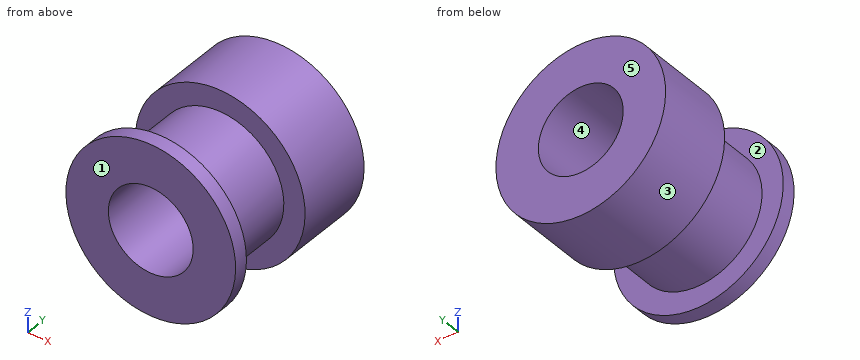
from build123d import *

# Parameters (mm, degrees)
SKETCH_1_R          = 8
EXTRUDE_1_DEPTH     = 1.35
SKETCH_4_R          = 6
EXTRUDE_3_DEPTH     = 7.3
EXTRUDE_START       = 8.65
SKETCH_1_3_R        = 8
EXTRUDE_4_DEPTH     = 7.35
SKETCH_5_R          = 4
CUT_EXTRUDE_1_DEPTH = 20.595917942


with BuildPart() as part:
    # 草图1 → 凸台-拉伸1 (new body)
    with BuildSketch(Plane(origin=(0, 0, 0), x_dir=(1, 0, 0), z_dir=(0, 1, 0))):
        with Locations(Location((0, 0, 0), (0, 0, 90))):
            Circle(SKETCH_1_R)
    extrude(amount=EXTRUDE_1_DEPTH)

    # 草图4 → 凸台-拉伸3 (add)
    with BuildSketch(Plane(origin=(0, 1.35, 0), x_dir=(1, 0, 0), z_dir=(0, 1, 0))):
        with Locations(Location((0, 0, 0), (0, 0, 270))):
            Circle(SKETCH_4_R)
    extrude(amount=EXTRUDE_3_DEPTH)

    # 草图1<3> → 凸台-拉伸4 (add)
    with BuildSketch(Plane(origin=(0, 0, 0), x_dir=(1, 0, 0), z_dir=(0, 1, 0)).offset(EXTRUDE_START)):
        with Locations(Location((0, 0, 0), (0, 0, 90))):
            Circle(SKETCH_1_3_R)
    extrude(amount=EXTRUDE_4_DEPTH)

    # 草图5 → 切除-拉伸1 (cut, through all)
    with BuildSketch(Plane.XZ):
        with Locations(Location((0, 0, 0), (0, 0, 270))):
            Circle(SKETCH_5_R)
    extrude(amount=-CUT_EXTRUDE_1_DEPTH, mode=Mode.SUBTRACT)


solid = part.part
Read the model definition and answer for the solid it produces. Units are mm, in the model's axes. Face numbers are marked on the shaded views. A direction names the side the tool comes from. Round coordinates to 2 decimals unless told otherwise and drop trailing zeros. Write each loop counter-clockwise with the first axis right and the second up, starting at its lowest first coordinate (ties: lowest second). Pieces come first, ordered by that corner, then holes. Notation, with made-up numbers: M -7,89.25 L 22,89.25 A20 cw 22,105.25 Z; hole C 17,21.25 d4. An arc over 180 degrees is marked long. Use a Markdown table: item, result.
1) The part is cut by section C-C (y = 1). Write down the section's boundary in (x, z).
Answers follow:
| item | result |
|---|---|
| outline | C 0,0 d16; hole C 0,0 d8 |
2) A tool of negligible diameter and unlimited length cuts with its end or side. For the marked faces 1 and 2, from which of +Z, -Z, +X, -X, +Y, -Y can it reach the whole face along a straight path? Write none if from no direction.
Answers follow:
| item | result |
|---|---|
| face 1 | +Z, -Z, +X, -X, -Y |
| face 2 | none |
3) The part is cut by section A-A (x = 0). Write down the section's boundary in (y, z).
Answers follow:
| item | result |
|---|---|
| outline | M 0,-8 L 1.35,-8 L 1.35,-6 L 8.65,-6 L 8.65,-8 L 16,-8 L 16,-4 L 0,-4 Z; M 0,4 L 16,4 L 16,8 L 8.65,8 L 8.65,6 L 1.35,6 L 1.35,8 L 0,8 Z |
4) The part is cut by section D-D (x = 5.5). Write down the section's boundary in (y, z).
Answers follow:
| item | result |
|---|---|
| outline | M 0,-5.81 L 1.35,-5.81 L 1.35,-2.4 L 8.65,-2.4 L 8.65,-5.81 L 16,-5.81 L 16,5.81 L 8.65,5.81 L 8.65,2.4 L 1.35,2.4 L 1.35,5.81 L 0,5.81 Z |
5) The part is cut by section B-B (z = 0). Write down the section's boundary in (x, y).
Answers follow:
| item | result |
|---|---|
| outline | M -8,0 L -4,0 L -4,16 L -8,16 L -8,8.65 L -6,8.65 L -6,1.35 L -8,1.35 Z; M 4,0 L 8,0 L 8,1.35 L 6,1.35 L 6,8.65 L 8,8.65 L 8,16 L 4,16 Z |
6) Flat-ended cylindrical pins translate along their axes: pin 1 (1.5 mm diameter, centred on x = 5.5, y = 10, fed in from -Z); pin 2 (1.5 mm diameter, centred on x = -6, y = 4, fed in from -Z); pin 3 (1.5 mm diameter, centred on x = -2.5, y = 2, fed in from +Z). Find the tip coordinate at first contact, or state that the pin passes through.
Answers follow:
| item | result |
|---|---|
| pin 1 | stops at z = -6.44 |
| pin 2 | stops at z = -2.9 |
| pin 3 | stops at z = 7.71 |
7) Straight lines are drawn through the part: line 1 along Y through (x, z) = (2.75, 6); line 2 along X through (y, z) = (7.75, 0); line 3 along X through (y, z) = (8.75, 0). For each, find the intervals that lie inside material, in ascending order. Write a range as [from, to].
Answers follow:
| item | result |
|---|---|
| line 1 | y = [0, 1.35], [8.65, 16] |
| line 2 | x = [-6, -4], [4, 6] |
| line 3 | x = [-8, -4], [4, 8] |
8) For a pull along X with two mould halves and no side action, classify the marked faces 3, 4 and 5 as pulls with the +X half, pulls with the -X half, needs draft (parallel to the pull), parting line crosses it, or undercut.
Answers follow:
| item | result |
|---|---|
| face 3 | parting line crosses it |
| face 4 | undercut |
| face 5 | needs draft |
